The listing builds one solid part. Answer for the finished solid, in the listing's coordinates (mm). A direction names the side the tool comes from. Give positions to 0.01 mm unless a question says otherwise; leave off trailing zeros. Loops run counter-clockwise (first coordinate to the right, second up) from the corner with the lowest first, then second, coordinate; pieces in that order, holes last. Notation, with made-up numbers: M -40,56 L 2,56 A22 ccw 2,64 Z; hole C 17.25,45.5 d6. An arc over 180 degrees is marked long. Use one line per item in the form item = value. Start each with the question number.
1. The part is cut by section B-B (z = -14.5). Write down the section's boundary in (x, y), and give its area (3 significant figures).
2. The mould has two halves that part along X. Classify faces 1 (the face through (3.92, -1.42, -22)), 2 (the face through (-6, -1.3, 7.3)), 3 (the face through (1.708, 3.014, 9.86)): released by +X, released by -X, zero draft, split by the parting line, or undercut.
3. For faces 4 (the face through (-7.52, -1.15, 16.77)), 5 (the face through (0, 0, 0)), 6 (the face through (5.723, -1.802, -10.846)), determine the directions among +Z, -Z, +X, -X, +Y, -Y from which every point of the face is accessible in a straight line to the end or side of a thin tool.
4. Each of these flat-tipped pins is pushed along its axis until it touches: pin 1 Ø3 at (y, z) = (1.5, 13) entering from +X; pin 2 Ø6 at (x, z) = (-1.5, -29.5) entering from -Y; pin 3 Ø3 at (x, z) = (-6.5, 0.5) entering from -Y. Where does it stop, or does it pass through?
5. Straight lines are drawn through the part: line 1 (Z direction, x = 7.55, y = 0); line 2 (Z direction, x = -4.25, y = 0.5); line 3 (Y direction, x = 4.2, z = 14). For each, find the intervals that lie inside material, in ascending order. Write a range as from..to.
6. The part is cut by section A-A (y = 164). Write down the section's boundary in (x, z).
from build123d import *

# Parameters (mm, degrees)
SKETCH1_R                = 9
BOSS_EXTRUDE1_DEPTH      = 20
BOSS_EXTRUDE3_REACH      = 204.69
BOSS_EXTRUDE3_END_RADIUS = 9
SKETCH6_R                = 4
CUT_EXTRUDE1_DEPTH       = 9
CUT_EXTRUDE1_DEPTH_BACK  = 9
SKETCH8_R                = 1.55
SKETCH11_R               = 6
BOSS_EXTRUDE12_DEPTH     = 22
SKETCH12_R               = 4
BOSS_EXTRUDE13_DEPTH     = 8
BOSS_EXTRUDE14_DEPTH     = 7
SKETCH14_R               = 1.55
CUT_EXTRUDE2_DEPTH       = 6.1
SKETCH15_R               = 3
BOSS_EXTRUDE15_DEPTH     = 10
CUT_EXTRUDE5_START       = 9
SKETCH16_R               = 3
CUT_EXTRUDE5_DEPTH       = 3
CUT_EXTRUDE6_START       = -6
SKETCH16_2_R             = 3
CUT_EXTRUDE6_DEPTH       = 3


with BuildPart() as part:
    # Sketch1 → Boss-Extrude1 (new body)
    with BuildSketch(Plane.XY):
        Circle(SKETCH1_R)
        Polygon((0, 4), (3.464101615, 2), (3.464101615, -2), (0, -4), (-3.464101615, -2), (-3.464101615, 2), align=None, mode=Mode.SUBTRACT)
    extrude(amount=BOSS_EXTRUDE1_DEPTH)

    # Boss-Extrude3: up to this cylinder (the profile starts outside it)
    boss_extrude3_end = Plane(origin=(0, 0, 10), z_dir=(0, 0, -1)) * Cylinder(BOSS_EXTRUDE3_END_RADIUS, 428.38, mode=Mode.PRIVATE)
    # Sketch6 → Boss-Extrude3 (add, up to the surface)
    with BuildSketch(Plane(origin=(0, 192.5, 0), x_dir=(1, 0, 0), z_dir=(0, 1, 0)), mode=Mode.PRIVATE) as boss_extrude3_sk1:
        with Locations(Location((0, -10, 0), (0, 0, 270))):
            Circle(SKETCH6_R)
    boss_extrude3_tool1 = extrude(boss_extrude3_sk1.sketch, amount=-BOSS_EXTRUDE3_REACH, mode=Mode.PRIVATE) - boss_extrude3_end
    add(boss_extrude3_tool1.solids().sort_by_distance((0, 192.5, 10))[0])

    # Sketch8 → Cut-Extrude1 (cut, two sides: drawn at the far end of the back side and taken through both)
    with BuildSketch(Plane.ZY.offset(-CUT_EXTRUDE1_DEPTH_BACK)):
        with Locations(Location((6, 0, 0), (0, 0, 180))):
            Circle(SKETCH8_R)
        with Locations(Location((14, 0, 0), (0, 0, 180))):
            Circle(SKETCH8_R)
    extrude(amount=CUT_EXTRUDE1_DEPTH + CUT_EXTRUDE1_DEPTH_BACK, mode=Mode.SUBTRACT)

    # Sketch11 → Boss-Extrude12 (add)
    with BuildSketch(Plane(origin=(0, 0, 0), x_dir=(-1, 0, 0), z_dir=(0, 0, -1))):
        with Locations(Location((0, 0, 0), (0, 0, 180))):
            Circle(SKETCH11_R)
    extrude(amount=BOSS_EXTRUDE12_DEPTH)

    # Sketch12 → Boss-Extrude13 (add)
    with BuildSketch(Plane(origin=(0, 0, -22), x_dir=(-1, 0, 0), z_dir=(0, 0, -1))):
        Circle(SKETCH12_R)
    extrude(amount=BOSS_EXTRUDE13_DEPTH)

    # Sketch13 → Boss-Extrude14 (add)
    with BuildSketch(Plane(origin=(0, 0, -30), x_dir=(-1, 0, 0), z_dir=(0, 0, -1))):
        Polygon((1.75, 3.031088913), (-1.75, 3.031088913), (-3.5, 0), (-1.75, -3.031088913), (1.75, -3.031088913), (3.5, 0), align=None)
    extrude(amount=BOSS_EXTRUDE14_DEPTH)

    # Sketch14 → Cut-Extrude2 (cut)
    with BuildSketch(Plane(origin=(2.625, -1.515544457, 0), x_dir=(0, 0, -1), z_dir=(0.8660254037844379, -0.5000000000000011, 0))):
        with Locations(Location((33.5, 0, 0), (0, 0, 90))):
            Circle(SKETCH14_R)
    extrude(amount=-CUT_EXTRUDE2_DEPTH, mode=Mode.SUBTRACT)

    # Sketch15 → Boss-Extrude15 (add)
    with BuildSketch(Plane(origin=(0, 0, -37), x_dir=(-1, 0, 0), z_dir=(0, 0, -1))):
        Circle(SKETCH15_R)
    extrude(amount=BOSS_EXTRUDE15_DEPTH)

    # Sketch16 → Cut-Extrude5 (cut)
    with BuildSketch(Plane.ZY.offset(CUT_EXTRUDE5_START)):
        with Locations((6, 0)):
            Circle(SKETCH16_R)
        with Locations((14, 0)):
            Circle(SKETCH16_R)
    extrude(amount=-CUT_EXTRUDE5_DEPTH, mode=Mode.SUBTRACT)

    # Sketch16_2 → Cut-Extrude6 (cut)
    with BuildSketch(Plane.ZY.offset(CUT_EXTRUDE6_START)):
        with Locations((6, 0)):
            Circle(SKETCH16_2_R)
        with Locations((14, 0)):
            Circle(SKETCH16_2_R)
    extrude(amount=-CUT_EXTRUDE6_DEPTH, mode=Mode.SUBTRACT)


solid = part.part
Derived:
q1.outline = C 0,0 d12
q1.area = 113 mm2
q2.face_1 = zero draft
q2.face_2 = released by -X
q2.face_3 = undercut
q3.face_4 = -X
q3.face_5 = +Z
q3.face_6 = -Z
q4.pin_1 = 8.84
q4.pin_2 = -4
q4.pin_3 = -7.48
q5.line_1 = 0..3, 9..11, 17..20
q5.line_2 = -22..4.53, 7.47..12.53, 15.47..20
q5.line_3 = -7.96..-1.55, 1.55..7.96
q6.outline = C 0,10 d8
